Verification items for the finished model (mm, model axes). A direction names the side the tool comes from. Give positions to 0.01 mm unless a question says otherwise; leave off trailing zeros. Order: outer loops, then holes, each group sorted by start corner. A loop starts at its lowest first (then second) coordinate and runs counter-clockwise, first axis right, second up. Notation, with made-up numbers: (29.25, -16.5) -> (46.25, -16.5) arc R17 cw to (46.25, 1.5) -> close; hole circle Ø5 at (3, 9). An arc over 180 degrees is marked (long way). Write each question's results on one line, items separated by ' | '. Start each with the question number.
1. Cross-section at D-D, the plane y = 18. Enter the section's corners in (x, z).
2. Depth check by flat-ended pin: pin 1 Ø5 at (x, y) = (63.5, 24.5) entering from +Z; pin 2 Ø4 at (y, z) = (21.5, 60) entering from +X; pin 3 Ø1.2 at (x, z) = (38.5, 66.5) entering from +Y; pin 4 Ø4.5 at (x, y) = (39.5, 29) entering from -Z. Enter the tip coordinate at first touch or a pass-through.
3. Set-up check for faces 5 (the face through (39, 43.3, 66)), 6 (the face through (80, 25.2, 67)), 7 (the face through (79, 18, 66)): record each of +Z, -Z, +X, -X, +Y, -Y from which the full face is reachable in a straight line by a thin tool's end or side.
4. Cross-section at A-A, the plane y = 26. Enter the section's corners in (x, z), then the cut area to 3 significant figures.
5. Mould release check, pull along X, two halves, no side actions. Record for faces 1 (the face through (84, 23, 74)), 2 (the face through (39, 23, 67)), 3 (the face through (36, 24, 74)), 4 (the face through (81, 43.3, 66)): +X half, -X half, draft (parallel to the pull), parting line (faces both ways), or undercut.
6. Cross-section at C-C, the plane x = 42.5. Enter the section's corners in (y, z), then the cut area to 3 significant figures.
7. Material ranges on L1, parallel to Y at x = 80, z = 72.25; L2, parallel to Y at x = 64, z = 74; L3, parallel to X at y = 16, z = 67.5, recorded low to high. Write a range as from..to.
from build123d import *

# Parameters (mm, degrees)
SKETCH2_W                = 200
SKETCH2_H                = 150
BOSS_EXTRUDE1_DEPTH      = 80
FILLET1_R                = 10
SHELL1_T                 = -2
SHELL1_THICKNESS_2_DEPTH = 13
SKETCH5_W                = 36.5
SKETCH5_H                = 27.5
CUT_EXTRUDE1_DEPTH       = 2
BOSS_EXTRUDE2_DEPTH      = 16
SKETCH7_W                = 36.5
SKETCH7_H                = 27.5
CUT_EXTRUDE2_DEPTH       = 2
BOSS_EXTRUDE3_DEPTH      = 16
SKETCH10_W               = 36.5
SKETCH10_H               = 27.5
CUT_EXTRUDE4_DEPTH       = 2
BOSS_EXTRUDE4_DEPTH      = 16
SKETCH13_W               = 2
SKETCH13_H               = 4
CUT_EXTRUDE5_DEPTH       = 2
BOSS_EXTRUDE5_DEPTH      = 13.5
SKETCH15_W               = 10.5
SKETCH15_H               = 7.1
CUT_EXTRUDE6_DEPTH       = 4
CUT_EXTRUDE8_REACH       = 150.408
SKETCH20_R               = 8
SPLIT1_SURFACE_1_BACK    = 263.488
SPLIT1_SURFACE_1_DEPTH   = 526.976
SPLIT1_SURFACE_2_BACK    = 263.488
SPLIT1_SURFACE_2_DEPTH   = 526.976
SPLIT2_SURFACE_3_BACK    = 263.488
SPLIT2_SURFACE_3_DEPTH   = 526.976
SPLIT2_SURFACE_4_BACK    = 263.488
SPLIT2_SURFACE_4_DEPTH   = 526.976


with BuildPart() as part:
    # Sketch2 → Boss-Extrude1 (new body)
    with BuildSketch(Plane(origin=(0, 0, 0), x_dir=(1, 0, 0), z_dir=(0, 1, 0))):
        Rectangle(SKETCH2_W, SKETCH2_H)
    extrude(amount=BOSS_EXTRUDE1_DEPTH)

    # Fillet1
    fillet1_edges = [part.edges().sort_by_distance(p)[0] for p in [
        (100, 40, 75),
        (-100, 40, 75),
        (-100, 40, -75),
        (100, 40, -75),
    ]]
    fillet(fillet1_edges, radius=FILLET1_R)

    # Shell1
    shell1_openings = [part.faces().sort_by_distance(p)[0] for p in [
        (0, 80, 0),
    ]]
    offset(amount=SHELL1_T, openings=shell1_openings, kind=Kind.INTERSECTION)

    # Shell1 thickness 2 face (on inner face of the shell) → Shell1 thickness 2 (add)
    with BuildSketch(Plane(origin=(0, 2, 0), x_dir=(0, 0, -1), z_dir=(0, -1, 0))):
        with BuildLine():
            ThreePointArc((73, -90), (70.656854249, -95.656854249), (65, -98))
            Line((65, -98), (-65, -98))
            ThreePointArc((-65, -98), (-70.656854249, -95.656854249), (-73, -90))
            Line((-73, -90), (-73, 90))
            ThreePointArc((-73, 90), (-70.656854249, 95.656854249), (-65, 98))
            Line((-65, 98), (65, 98))
            ThreePointArc((65, 98), (70.656854249, 95.656854249), (73, 90))
            Line((73, 90), (73, -90))
        make_face()
    extrude(amount=-SHELL1_THICKNESS_2_DEPTH)

    # Sketch5 → Cut-Extrude1 (cut)
    with BuildSketch(Plane.XY.offset(75)):
        with Locations((0, 30.75)):
            Rectangle(SKETCH5_W, SKETCH5_H)
        Polygon((-18.25, 43.5), (-19.75, 44.366025404), (-19.75, 41.633974596), (-18.25, 42.5), align=None)
        Polygon((-19.75, 19.866025404), (-18.25, 19), (-18.25, 18), (-19.75, 17.133974596), align=None)
        Polygon((19.75, 17.133974596), (19.75, 19.866025404), (18.25, 19), (18.25, 18), align=None)
        Polygon((19.75, 41.633974596), (18.25, 42.5), (18.25, 43.5), (19.75, 44.366025404), align=None)
    extrude(amount=-CUT_EXTRUDE1_DEPTH, mode=Mode.SUBTRACT)

    # Sketch6 → Boss-Extrude2 (add)
    with BuildSketch(Plane(origin=(0, 0, 73), x_dir=(-1, 0, 0), z_dir=(0, 0, -1))):
        Polygon((18.25, 15), (21.25, 15), (21.25, 47.5), (18.25, 47.5), (18.25, 43.5), (19.75, 44.366025404), (19.75, 41.633974596), (18.25, 42.5), (18.25, 19), (19.75, 19.866025404), (19.75, 17.133974596), (18.25, 18), align=None)
        Polygon((-21.25, 47.5), (-21.25, 15), (-18.25, 15), (-18.25, 18), (-19.75, 17.133974596), (-19.75, 19.866025404), (-18.25, 19), (-18.25, 42.5), (-19.75, 41.633974596), (-19.75, 44.366025404), (-18.25, 43.5), (-18.25, 47.5), align=None)
    extrude(amount=BOSS_EXTRUDE2_DEPTH)

    # Sketch7 → Cut-Extrude2 (cut)
    with BuildSketch(Plane(origin=(100, 0, 0), x_dir=(0, 0, -1), z_dir=(1, 0, 0))):
        with Locations((0, 30.75)):
            Rectangle(SKETCH7_W, SKETCH7_H)
        Polygon((-18.25, 43.5), (-19.75, 44.366025404), (-19.75, 41.633974596), (-18.25, 42.5), align=None)
        Polygon((-19.75, 19.866025404), (-18.25, 19), (-18.25, 18), (-19.75, 17.133974596), align=None)
        Polygon((19.75, 17.133974596), (19.75, 19.866025404), (18.25, 19), (18.25, 18), align=None)
        Polygon((19.75, 41.633974596), (18.25, 42.5), (18.25, 43.5), (19.75, 44.366025404), align=None)
    extrude(amount=-CUT_EXTRUDE2_DEPTH, mode=Mode.SUBTRACT)

    # Sketch8 → Boss-Extrude3 (add)
    with BuildSketch(Plane.ZY.offset(-98)):
        Polygon((-21.25, 47.5), (-18.25, 47.5), (-18.25, 43.5), (-19.75, 44.366025404), (-19.75, 41.633974596), (-18.25, 42.5), (-18.25, 19), (-19.75, 19.866025404), (-19.75, 17.133974596), (-18.25, 18), (-18.25, 15), (-21.25, 15), align=None)
        Polygon((19.75, 44.366025404), (18.25, 43.5), (18.25, 47.5), (21.25, 47.5), (21.25, 15), (18.25, 15), (18.25, 18), (19.75, 17.133974596), (19.75, 19.866025404), (18.25, 19), (18.25, 42.5), (19.75, 41.633974596), align=None)
    extrude(amount=BOSS_EXTRUDE3_DEPTH)

    # Sketch10 → Cut-Extrude4 (cut)
    with BuildSketch(Plane.ZY.offset(100)):
        with Locations((0, 30.75)):
            Rectangle(SKETCH10_W, SKETCH10_H)
        Polygon((-18.25, 43.5), (-19.75, 44.366025404), (-19.75, 41.633974596), (-18.25, 42.5), align=None)
        Polygon((-19.75, 19.866025404), (-18.25, 19), (-18.25, 18), (-19.75, 17.133974596), align=None)
        Polygon((19.75, 17.133974596), (19.75, 19.866025404), (18.25, 19), (18.25, 18), align=None)
        Polygon((19.75, 41.633974596), (18.25, 42.5), (18.25, 43.5), (19.75, 44.366025404), align=None)
    extrude(amount=-CUT_EXTRUDE4_DEPTH, mode=Mode.SUBTRACT)

    # Sketch11 → Boss-Extrude4 (add)
    with BuildSketch(Plane(origin=(-98, 0, 0), x_dir=(0, 0, -1), z_dir=(1, 0, 0))):
        Polygon((-18.25, 47.5), (-21.25, 47.5), (-21.25, 15), (-18.25, 15), (-18.25, 18), (-19.75, 17.133974596), (-19.75, 19.866025404), (-18.25, 19), (-18.25, 42.5), (-19.75, 41.633974596), (-19.75, 44.366025404), (-18.25, 43.5), align=None)
        Polygon((19.75, 44.366025404), (18.25, 43.5), (18.25, 47.5), (21.25, 47.5), (21.25, 15), (18.25, 15), (18.25, 18), (19.75, 17.133974596), (19.75, 19.866025404), (18.25, 19), (18.25, 42.5), (19.75, 41.633974596), align=None)
    extrude(amount=BOSS_EXTRUDE4_DEPTH)

    # Sketch13 → Cut-Extrude5 (cut)
    with BuildSketch(Plane.XY.offset(75)):
        with Locations((40, 38.3)):
            Rectangle(SKETCH13_W, SKETCH13_H)
        Polygon((79, 40.3), (41, 40.3), (41, 36.3), (41, 25.2), (41, 21.2), (79, 21.2), (79, 25.2), (79, 36.3), align=None)
        with Locations((80, 38.3)):
            Rectangle(SKETCH13_W, SKETCH13_H)
        with Locations((40, 23.2)):
            Rectangle(SKETCH13_W, SKETCH13_H)
        with Locations((80, 23.2)):
            Rectangle(SKETCH13_W, SKETCH13_H)
    extrude(amount=-CUT_EXTRUDE5_DEPTH, mode=Mode.SUBTRACT)

    # Sketch14 → Boss-Extrude5 (add)
    with BuildSketch(Plane(origin=(0, 0, 73), x_dir=(-1, 0, 0), z_dir=(0, 0, -1))):
        Polygon((-79, 43.3), (-83, 43.3), (-83, 15), (-79, 15), (-79, 21.2), (-81, 21.2), (-81, 25.2), (-79, 25.2), (-79, 36.3), (-81, 36.3), (-81, 40.3), (-79, 40.3), align=None)
        Polygon((-39, 40.3), (-41, 40.3), (-41, 43.3), (-37, 43.3), (-37, 15), (-41, 15), (-41, 21.2), (-39, 21.2), (-39, 25.2), (-41, 25.2), (-41, 36.3), (-39, 36.3), align=None)
    extrude(amount=BOSS_EXTRUDE5_DEPTH)

    # Sketch15 → Cut-Extrude6 (cut)
    with BuildSketch(Plane.ZY.offset(-37)):
        with Locations((66.75, 30.75)):
            Rectangle(SKETCH15_W, SKETCH15_H)
    extrude(amount=-CUT_EXTRUDE6_DEPTH, mode=Mode.SUBTRACT)

    # Sketch18 → Cut-Revolve1 (revolve, cut)
    with BuildSketch(Plane(origin=(0, 0, 0), x_dir=(0, 0, -1), z_dir=(1, 0, 0)), mode=Mode.PRIVATE) as cut_revolve1_sk:
        Polygon((-42.5, 0), (-70, 0), (-47.5, 10), (-42.5, 10), align=None)
    revolve(cut_revolve1_sk.sketch.rotate(Axis((0, 0, 0), (0, 1, 0)), 180), axis=Axis((0, 0, 0), (0, 1, 0)), mode=Mode.SUBTRACT)

    # Cut-Extrude8: up to this face of the body (flat: up to its plane)
    cut_extrude8_end = Plane(part.part.faces().sort_by_distance((-0.230072279, 15, -0.475589226))[0])
    # Sketch20 → Cut-Extrude8 (cut, up to the picked face)
    with BuildSketch(Plane.XZ, mode=Mode.PRIVATE) as cut_extrude8_sk1:
        with Locations(Location((0, -42.5, 0), (0, 0, 270))):
            Circle(SKETCH20_R)
    cut_extrude8_tool1 = split(extrude(cut_extrude8_sk1.sketch, amount=-CUT_EXTRUDE8_REACH, mode=Mode.PRIVATE), bisect_by=cut_extrude8_end, keep=Keep.BOTH, mode=Mode.PRIVATE)
    add(cut_extrude8_tool1.solids().sort_by(Axis((0, 0, -42.5), (0, 1, 0)))[0], mode=Mode.SUBTRACT)


with BuildPart() as body_2:
    # Split1: the piece behind the surface
    add(part.part)
    # Split1 surface: a surface, the sketch's curves swept straight by 526.976 mm
    with BuildLine(Plane.XY.offset(75).offset(-SPLIT1_SURFACE_1_BACK), mode=Mode.PRIVATE) as split1_surface_1_path:
        Line((36, 49.5), (84, 49.5))
        Line((84, 49.5), (84, 12))
        Line((84, 12), (36, 12))
        Line((36, 12), (36, 49.5))
    split1_surface_1 = Shell.extrude(split1_surface_1_path.wire(), (0 * SPLIT1_SURFACE_1_DEPTH, 0 * SPLIT1_SURFACE_1_DEPTH, 1 * SPLIT1_SURFACE_1_DEPTH))
    split(bisect_by=split1_surface_1, keep=Keep.BOTTOM)


with BuildPart() as part_1:
    add(part.part)

    # Split1: split by a surface, the side it looks to stays
    # Split1 surface: a surface, the sketch's curves swept straight by 526.976 mm
    with BuildLine(Plane.XY.offset(75).offset(-SPLIT1_SURFACE_2_BACK), mode=Mode.PRIVATE) as split1_surface_2_path:
        Line((36, 49.5), (84, 49.5))
        Line((84, 49.5), (84, 12))
        Line((84, 12), (36, 12))
        Line((36, 12), (36, 49.5))
    split1_surface_2 = Shell.extrude(split1_surface_2_path.wire(), (0 * SPLIT1_SURFACE_2_DEPTH, 0 * SPLIT1_SURFACE_2_DEPTH, 1 * SPLIT1_SURFACE_2_DEPTH))
    split(bisect_by=split1_surface_2, keep=Keep.TOP)


with BuildPart() as body_3:
    # Split2: the piece behind the surface
    add(body_2.part)
    # Split2 surface: a surface, the sketch's curves swept straight by 526.976 mm
    with BuildLine(Plane(origin=(0, 15, 0), x_dir=(1, 0, 0), z_dir=(0, 1, 0)).offset(-SPLIT2_SURFACE_3_BACK), mode=Mode.PRIVATE) as split2_surface_3_path:
        Line((36, -75), (84, -75))
        Line((84, -75), (84, -55))
        Line((84, -55), (36, -55))
        Line((36, -55), (36, -75))
    split2_surface_3 = Shell.extrude(split2_surface_3_path.wire(), (0 * SPLIT2_SURFACE_3_DEPTH, 1 * SPLIT2_SURFACE_3_DEPTH, 0 * SPLIT2_SURFACE_3_DEPTH))
    split(bisect_by=split2_surface_3, keep=Keep.BOTTOM)


with BuildPart() as body_2_1:
    add(body_2.part)

    # Split2: split by a surface, the side it looks to stays
    # Split2 surface: a surface, the sketch's curves swept straight by 526.976 mm
    with BuildLine(Plane(origin=(0, 15, 0), x_dir=(1, 0, 0), z_dir=(0, 1, 0)).offset(-SPLIT2_SURFACE_4_BACK), mode=Mode.PRIVATE) as split2_surface_4_path:
        Line((36, -75), (84, -75))
        Line((84, -75), (84, -55))
        Line((84, -55), (36, -55))
        Line((36, -55), (36, -75))
    split2_surface_4 = Shell.extrude(split2_surface_4_path.wire(), (0 * SPLIT2_SURFACE_4_DEPTH, 1 * SPLIT2_SURFACE_4_DEPTH, 0 * SPLIT2_SURFACE_4_DEPTH))
    split(bisect_by=split2_surface_4, keep=Keep.TOP)


solid = body_2_1.part
Results below:
1) outline: (36, 73) -> (37, 73) -> (37, 59.5) -> (41, 59.5) -> (41, 73) -> (79, 73) -> (79, 59.5) -> (83, 59.5) -> (83, 73) -> (84, 73) -> (84, 75) -> (36, 75) -> close
2) pin 1: passes through | pin 2: stops at x = 83 | pin 3: stops at y = 43.3 | pin 4: stops at z = 59.5
3) face 5: -Z, +X, -X, +Y | face 6: +Z, -Z | face 7: -Z, +Y
4) outline: (36, 73) -> (37, 73) -> (37, 59.5) -> (41, 59.5) -> (41, 75) -> (36, 75) -> close; (79, 59.5) -> (83, 59.5) -> (83, 73) -> (84, 73) -> (84, 75) -> (79, 75) -> close | area: 128 mm²
5) face 1: +X half | face 2: undercut | face 3: -X half | face 4: draft
6) outline: (12, 55) -> (15, 55) -> (15, 73) -> (21.2, 73) -> (21.2, 75) -> (12, 75) -> close; (40.3, 73) -> (49.5, 73) -> (49.5, 75) -> (40.3, 75) -> close | area: 90.8 mm²
7) L1: y = 12..21.2, 25.2..36.3, 40.3..43.3 | L2: y = 12..21.2, 40.3..49.5 | L3: x = 37..41, 79..83
